Could you check a few things on this model? Use its own coordinates, in mm. A direction names the side the tool comes from. Give positions to 0.01 mm unless a question says otherwise; leave off trailing zeros. Write each loop counter-clockwise with the first axis right and the second up, starting at its lowest first coordinate (ties: lowest second). Pieces come first, ordered by that corner, then holes. Notation, with made-up numbers: M 62.5,-26.5 L 106.5,-26.5 A13 cw 106.5,-1.5 Z; hole C 41,75.25 d8. An arc over 180 degrees is marked long. One line per item, written item: value.
```python
from build123d import *

# Parameters (mm, degrees)
EXTRUDE_1210_DEPTH     = 7.95
CUT_EXTRUDE_1739_DEPTH = 87.052353761
FILLET_1_R             = 0.75
CUT_EXTRUDE_3017_DEPTH = 87.052353882
FILLET_START           = -9
FILLET_2_DEPTH         = 10
FILLET_3_DEPTH         = 10


with BuildPart() as part:
    # Эскиз1 → Extrude 1210 (new body)
    with BuildSketch(Plane.XY):
        with BuildLine():
            Line((-59.003125249, 1.5), (-59.003125249, 9))
            Line((-59.003125249, 9), (-67.003125249, 9))
            ThreePointArc((-67.003125249, 9), (-76.672665052, 5.982131454), (-82.909098969, -2))
            Line((-82.909098969, -2), (-84.909098969, -2))
            ThreePointArc((-84.909098969, -2), (-78.847334249, 7.709212734), (-68.047161318, 11.5))
            Line((-68.047161318, 11.5), (0, 11.5))
            Line((0, 11.5), (22.496874751, 11.5))
            ThreePointArc((22.496874751, 11.5), (32.529707481, 7.620316306), (37.34210733, -2))
            Line((37.34210733, -2), (35.34210733, -2))
            ThreePointArc((35.34210733, -2), (30.952642014, 5.874208829), (22.496874751, 9))
            Line((22.496874751, 9), (20.996874751, 9))
            Line((20.996874751, 9), (20.996874751, 1.5))
            ThreePointArc((20.996874751, 1.5), (-19.003125249, 6.931677052), (-59.003125249, 1.5))
        make_face()
    extrude(amount=-EXTRUDE_1210_DEPTH)

    # Эскиз5 → Cut-Extrude 1739 (cut, through all)
    with BuildSketch(Plane.XY):
        with BuildLine():
            Line((-56.503125249, 4), (-51.503125249, 4))
            ThreePointArc((-51.503125249, 4), (-50.503125249, 3), (-51.503125249, 2))
            Line((-51.503125249, 2), (-56.503125249, 2))
            ThreePointArc((-56.503125249, 2), (-57.503125249, 3), (-56.503125249, 4))
        make_face()
        with BuildLine():
            Line((18.496874751, 2), (13.496874751, 2))
            ThreePointArc((13.496874751, 2), (12.496874751, 3), (13.496874751, 4))
            Line((13.496874751, 4), (18.496874751, 4))
            ThreePointArc((18.496874751, 4), (19.496874751, 3), (18.496874751, 2))
        make_face()
    extrude(amount=-CUT_EXTRUDE_1739_DEPTH, mode=Mode.SUBTRACT)

    # Скругление1
    fillet_1_edges = [part.edges().sort_by_distance(p)[0] for p in [
        (-59.003125249, 1.5, -3.975),
        (-59.003125249, 9, -3.975),
        (20.996874751, 9, -3.975),
        (20.996874751, 1.5, -3.975),
        (-56.87546785, 2.071904645, -3.975),
        (18.869217353, 2.071904645, -3.975),
    ]]
    fillet(fillet_1_edges, radius=FILLET_1_R)

    # Эскиз3 → Cut-Extrude 3017 (cut, through all)
    with BuildSketch(Plane.XY):
        with BuildLine():
            Line((5.5, 11.5), (17.5, 11.5))
            ThreePointArc((17.5, 11.5), (11.5, 9.892304845), (5.5, 11.5))
        make_face()
    extrude(amount=-CUT_EXTRUDE_3017_DEPTH, mode=Mode.SUBTRACT)

    # Скругление2: read off the stored shape, not the designer's step
    # Скругление2 outline → Скругление2 (cut)
    with BuildSketch(Plane.XY.offset(FILLET_START)):
        with BuildLine():
            add(Edge.make_bspline(
                [(-83.594065856, -1.999999999), (-83.128693054, -2), (-82.805959239, -1.722499415), (-82.662093068, -1.382090449)],
                knots=[0.592824962, 0.592824962, 0.592824962, 0.592824962, 1, 1, 1, 1], degree=3, weights=[0.541566314, 0.5894209, 0.742232129, 1]))
            Line((-83.594065856, -1.999999999), (-82.909098969, -2))
            ThreePointArc((-82.909098969, -2), (-82.78861975, -1.689836505), (-82.662093068, -1.382090449))
        make_face()
        with BuildLine():
            add(Edge.make_bspline(
                [(-84.560958648, -0.690168037), (-84.749276161, -1.301091768), (-84.44037433, -1.999999997), (-83.594065856, -1.999999999)],
                knots=[0, 0, 0, 0, 0.592824962, 0.592824962, 0.592824962, 0.592824962], degree=3, weights=[1, 0.624703839, 0.47189261, 0.541566314]))
            ThreePointArc((-84.560958648, -0.690168037), (-84.747874965, -1.341669638), (-84.909098969, -2))
            Line((-84.909098969, -2), (-83.594065856, -1.999999999))
        make_face()
    extrude(amount=FILLET_2_DEPTH, mode=Mode.SUBTRACT)

    # Скругление3: read off the stored shape, not the designer's step
    # Скругление3 outline → Скругление3 (cut)
    with BuildSketch(Plane.XY.offset(FILLET_START)):
        with BuildLine():
            add(Edge.make_bspline(
                [(36.182438008, -1.999999999), (36.957978226, -1.999999999), (37.281497294, -1.380826049), (37.180278652, -0.809748442)],
                knots=[0.449797355, 0.449797355, 0.449797355, 0.449797355, 1, 1, 1, 1], degree=3, weights=[0.515263178, 0.479194979, 0.64077392, 1]))
            Line((36.182438008, -1.999999999), (37.34210733, -2))
            ThreePointArc((37.34210733, -2), (37.273182402, -1.40324412), (37.180278652, -0.809748442))
        make_face()
        with BuildLine():
            add(Edge.make_bspline(
                [(35.192752533, -1.204523772), (35.28524719, -1.624595617), (35.624720765, -1.999999999), (36.182438008, -1.999999999)],
                knots=[0, 0, 0, 0, 0.449797355, 0.449797355, 0.449797355, 0.449797355], degree=3, weights=[1, 0.70632831, 0.544749369, 0.515263178]))
            ThreePointArc((35.192752533, -1.204523772), (35.273622194, -1.601099256), (35.34210733, -2))
            Line((35.34210733, -2), (36.182438008, -1.999999999))
        make_face()
    extrude(amount=FILLET_3_DEPTH, mode=Mode.SUBTRACT)


solid = part.part
```
1) I'm going to push flat-ended pins straight in: pin 1 (2.5 mm diameter, centred on x = 15.5, z = -4.5, fed in from -Y); pin 2 (1.7 mm diameter, centred on y = 6, z = -5.5, fed in from +X); pin 3 (0.8 mm diameter, centred on x = 22, z = -3, fed in from -Y). Where does each tip first touch, or does it pass through?
Outcome:
pin 1: stops at y = 4
pin 2: stops at x = 34.71
pin 3: stops at y = 8.99
2) On a 3-axis mill with a long thin cutter (end or side, diameter ignored), from which of +Z, -Z, +X, -X, +Y, -Y can I reach the whole of each face in a straight line? I mean faces 1 (the face through (-32, 11.5, -4)), 2 (the face through (-63, 9, -4)). Say none if no direction works.
Outcome:
face 1: +Z, -Z, +X, -X, +Y
face 2: +Z, -Z, -Y
3) If we section it at B-B, the plane x = -32.5: Write out the boundary of the cut face in (y, z), then the cut area to 3 significant figures.
Outcome:
outline: M 6.32,-7.95 L 11.5,-7.95 L 11.5,0 L 6.32,0 Z
area: 41.2 mm^2
4) Please list where these lines run through material, in increasing order: L1, parallel to X at y = 2.25, z = -2.5; L2, parallel to X at y = 2.5, z = -2.75; L3, parallel to X at y = 0, z = -4. Write a range as from..to.
Outcome:
L1: x = -83.35..-80.57, -58.97..-57.47, 19.47..20.96, 33.9..36.29
L2: x = -83.21..-80.37, -59..-57.43, 19.42..21, 33.76..36.19
L3: x = -84.33..-82, 34.87..37.01
5) We'd pull the mould along X, two halves only. Please class faces 3 (the face through (-23, 8, 0)), 4 (the face through (-76.281, 6.245, -3.919)), 5 (the face through (-78.433, 8.03, -3.919)): pulls with the +X half, pulls with the -X half, needs draft (parallel to the pull), parting line crosses it, or undercut.
Outcome:
face 3: needs draft
face 4: undercut
face 5: pulls with the -X half
6) If we section it at A-A, the plane x = -62.5: Write out the boundary of the cut face in (y, z).
Outcome:
outline: M 9,-7.95 L 11.5,-7.95 L 11.5,0 L 9,0 Z
